Here's how the part is built. I have some questions about the finished solid (model axes, mm). Face numbers are marked on the shaded views. A direction names the side the tool comes from. Coordinates: 2 decimals unless noted, no trailing zeros. Write each loop counter-clockwise with the first axis right and the second up, starting at its lowest first coordinate (ties: lowest second). Pieces come first, ordered by that corner, then holes.
```python
from build123d import *

# Parameters (mm, degrees)
F1_DEPTH = 3.175
F3_DEPTH = 34.925
F5_DEPTH = 34.925
F7_DEPTH = 34.925


with BuildPart() as f1:
    # F0 (on Front) → F1 (new body)
    with BuildSketch(Plane.XZ):
        Polygon((0, 80.828254), (0, 0), (38.1, 0), (38.1, 80.828254), (38.1, 134.70979), (38.1, 189.66895), (0, 189.66895), (0, 134.70979), align=None)
        Polygon((-80.828254, 0), (0, 80.828254), (0, 134.70979), (-134.70979, 0), align=None)
        Polygon((38.1, 134.70979), (38.1, 80.828254), (118.928254, 0), (172.80979, 0), align=None)
    extrude(amount=F1_DEPTH)

    # F2 (on face) → F3 (join)
    with BuildSketch(Plane(origin=(0, 0, 0), x_dir=(-1, 0, 0), z_dir=(0, 1, 0))):
        Polygon((-38.1, 80.828254), (-38.1, 0), (-34.925, 0), (-34.925, 189.66895), (-38.1, 189.66895), (-38.1, 134.70979), align=None)
    extrude(amount=F3_DEPTH)

    # F4 (on face) → F5 (join)
    with BuildSketch(Plane(origin=(0, 0, 0), x_dir=(-1, 0, 0), z_dir=(0, 1, 0))):
        Polygon((-123.418382, 0), (-118.928254, 0), (-38.1, 80.828254), (-38.1, 85.318382), align=None)
    extrude(amount=F5_DEPTH)

    # F6 (on face) → F7 (join)
    with BuildSketch(Plane(origin=(0, 0, 0), x_dir=(-1, 0, 0), z_dir=(0, 1, 0))):
        Polygon((0, 80.828254), (80.828254, 0), (85.318382, 0), (0, 85.318382), align=None)
    extrude(amount=F7_DEPTH)


solid = f1.part
```
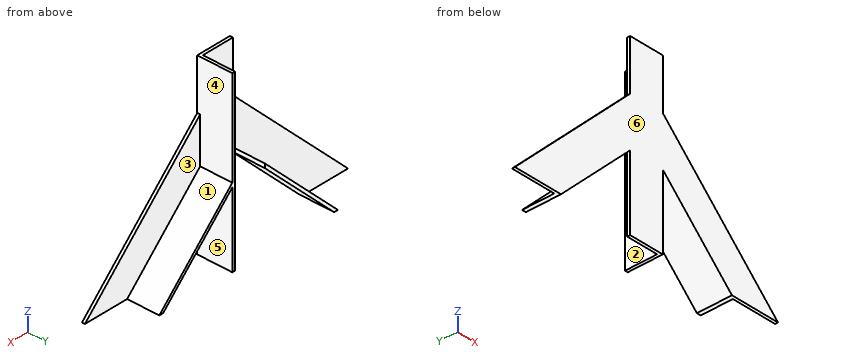
1) Imagine slicing it at D-D on z = 100.5. Please give me the cut outline in (x, y) (3 decimals), then the cut area to 3 significant figures.
Values follow:
outline: (-34.21, -3.175) - (72.31, -3.175) - (72.31, 0) - (38.1, 0) - (38.1, 34.925) - (34.925, 34.925) - (34.925, 0) - (-34.21, 0) - close
area: 449 mm2
2) Imagine slicing it at B-B on z = 18. Please give me the cut outline in (x, y) (3 decimals), then the cut area to 3 significant figures.
Values follow:
outline: (-116.71, -3.175) - (-62.828, -3.175) - (-62.828, 34.925) - (-67.318, 34.925) - (-67.318, 0) - (-116.71, 0) - close; (0, -3.175) - (38.1, -3.175) - (38.1, 34.925) - (34.925, 34.925) - (34.925, 0) - (0, 0) - close; (100.928, -3.175) - (154.81, -3.175) - (154.81, 0) - (105.418, 0) - (105.418, 34.925) - (100.928, 34.925) - close
area: 888 mm2
3) I need wall thicknesses on probe 1 along X at (y, z) = (23.5, 48) (3 decimals); probe 2 along X at (y, z) = (22, 26.5) (3 decimals); probe 3 along Y at (x, z) = (-37.5, 57.5) (3 decimals). Which ranges of each line are inside material? Lowest first, please.
Values follow:
probe 1: x = -37.318 to -32.828, 34.925 to 38.1, 70.928 to 75.418
probe 2: x = -58.818 to -54.328, 34.925 to 38.1, 92.428 to 96.918
probe 3: y = -3.175 to 0
4) On a 3-axis mill with a long thin cutter (end or side, diameter ignored), from which of +Z, -Z, +X, -X, +Y, -Y can I reach the whole of each face in a straight line? I mean the marked faces 4, 5 and 6. Say none if no direction works.
Values follow:
face 4: +Z, +X, +Y
face 5: -Z, +Y, -Y
face 6: +Z, -Z, +X, -X, -Y
5) Imagine slicing it at A-A on y = 15. Please give me the cut outline in (x, z) (3 decimals), then the cut area to 3 significant figures.
Values follow:
outline: (-85.318, 0) - (-80.828, 0) - (0, 80.828) - (0, 85.318) - close; (34.925, 0) - (38.1, 0) - (38.1, 80.828) - (118.928, 0) - (123.418, 0) - (38.1, 85.318) - (38.1, 189.669) - (34.925, 189.669) - close
area: 1,350 mm2
6) Imagine slicing it at C-C on x = 14. Please give me the cut outline in (y, z) (3 decimals), then the cut area to 3 significant figures.
Values follow:
outline: (-3.175, 0) - (0, 0) - (0, 189.669) - (-3.175, 189.669) - close
area: 602 mm2
7) We'd pull the mould along X, two halves only. Please class the marked faces 1, 2 and 3: pulls with the +X half, pulls with the -X half, needs draft (parallel to the pull), parting line crosses it, or undercut.
Values follow:
face 1: pulls with the +X half
face 2: undercut
face 3: needs draft
8) Will these pins go through, and if not, where does the flat tip stop? pin 1 (2 mm diameter, centred on y = 19.5, z = 84, fed in from +X); pin 2 (12 mm diameter, centred on x = -76.5, y = 20.5, fed in from +Z); pin 3 (10 mm diameter, centred on y = 8.5, z = 103, fed in from -X) (3 decimals).
Values follow:
pin 1: stops at x = 40.42
pin 2: stops at z = 14.82
pin 3: stops at x = 34.925
